Here's how the part is built. I have some questions about the finished solid (model axes, mm). Face numbers are marked on the shaded views. A direction names the side the tool comes from. Round coordinates to 2 decimals unless told otherwise and drop trailing zeros. Write each loop counter-clockwise with the first axis right and the second up, starting at its lowest first coordinate (ties: lowest second). Pieces come first, ordered by that corner, then holes. Notation, with made-up numbers: (31.5, -25) - (88.5, -25) arc R25 cw to (88.5, -13) - close; hole circle Ø6 at (-10, -21). An arc over 180 degrees is marked (long way). Write item = value, one per line. Start each with the question number.
Item 1: For P1, Ø4, axis at x = 25.5, y = -17, coming from the -Z side; P2, Ø3.5, axis at y = -20, z = 24.5, coming from the +X side; P3, Ø11.5, axis at x = 60, z = 27.5, coming from the -Y side; P4, Ø1.5, axis at y = -24, z = 17, coming from the +X side, each with a flat end and sliding along its axis, tell me the tip position at first contact or that it passes through.
Item 2: Thinking about a two-plate mould opening in X: for the marked faces 4, 5, 6 and 7, which applies, pulls with the +X half, pulls with the -X half, needs draft (parallel to the pull), parting line crosses it, or undercut?
Item 3: If we section it at D-D (z = 7.5): Please give me the cut outline in (x, y).
Item 4: If we section it at B-B (x = 31.71): Please give me the cut outline in (y, z).
Item 5: If we section it at C-C (y = -16.5): Please give me the cut outline in (x, z), and give its area (3 significant figures).
Item 6: If we section it at A-A (z = 19.17): Please give me the cut outline in (x, y).
Item 7: Which directions (+Z, -Z, +X, -X, +Y, -Y) give clear straight access to the entire face, cutting with the end or side of a thin tool? Please do the marked faces 1, 2 and 3.
Item 8: If I drill on line 1 along Z through (x, y) = (31.71, -8.75); line 2 along Y through (x, z) = (40, 13); line 3 along Y through (x, z) = (53, 5), over which ranges is the centre line in solid material (lowest first)? Write a range as [from, to].
```python
from build123d import *

# Parameters (mm, degrees)
F0_W     = 8.18
F0_H     = 38.16
F1_DEPTH = 25.3
F0_W_2   = 44.44
F0_R     = 6.47
F2_DEPTH = 22.4
F3_START = 2.94
F0_W_3   = 10.3
F3_DEPTH = 12.5


with BuildPart() as f1:
    # F0 (on Front) → F1 (new body)
    with BuildSketch(Plane.XZ):
        with Locations((4.09, 19.08)):
            Rectangle(F0_W, F0_H)
    extrude(amount=F1_DEPTH)

    # F0 (on Front) → F2 (join)
    with BuildSketch(Plane.XZ):
        with Locations((30.4, 19.08)):
            Rectangle(F0_W_2, F0_H)
        with Locations((31.71, 19.17)):
            Circle(F0_R, mode=Mode.SUBTRACT)
    extrude(amount=F2_DEPTH)

    # F0 (on Front) → F3 (join)
    with BuildSketch(Plane.XZ.offset(F3_START)):
        with Locations((57.77, 19.08)):
            Rectangle(F0_W_3, F0_H)
    extrude(amount=F3_DEPTH)


solid = f1.part
```
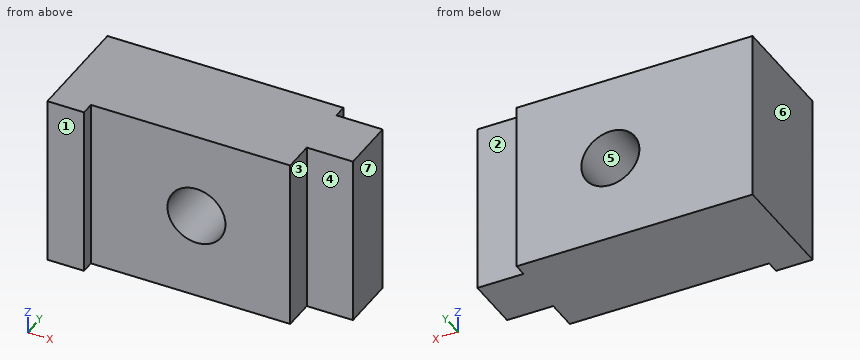
Reply:
q1.P1 = 0
q1.P2 = 52.62
q1.P3 = -15.44
q1.P4 = 8.18
q2.face_4 = needs draft
q2.face_5 = undercut
q2.face_6 = pulls with the -X half
q2.face_7 = pulls with the +X half
q3.outline = (0, -25.3) - (8.18, -25.3) - (8.18, -22.4) - (52.62, -22.4) - (52.62, -15.44) - (62.92, -15.44) - (62.92, -2.94) - (52.62, -2.94) - (52.62, 0) - (0, 0) - close
q4.outline = (-22.4, 0) - (0, 0) - (0, 12.7) - (-22.4, 12.7) - close; (-22.4, 25.64) - (0, 25.64) - (0, 38.16) - (-22.4, 38.16) - close
q5.outline = (0, 0) - (52.62, 0) - (52.62, 38.16) - (0, 38.16) - close; hole circle Ø12.94 at (31.71, 19.17)
q5.area = 1,880 mm2
q6.outline = (0, -25.3) - (8.18, -25.3) - (8.18, -22.4) - (25.24, -22.4) - (25.24, 0) - (0, 0) - close; (38.18, -22.4) - (52.62, -22.4) - (52.62, -15.44) - (62.92, -15.44) - (62.92, -2.94) - (52.62, -2.94) - (52.62, 0) - (38.18, 0) - close
q7.face_1 = +Z, -Z, +X, -X, -Y
q7.face_2 = +Z, -Z, +X, +Y
q7.face_3 = +Z, -Z, +X, -Y
q8.line_1 = [0, 12.7], [25.64, 38.16]
q8.line_2 = [-22.4, 0]
q8.line_3 = [-15.44, -2.94]
